The listing builds one solid part. Answer for the finished solid, in the listing's coordinates (mm). A direction names the side the tool comes from. Coordinates: 2 decimals unless noted, no trailing zeros. Loops run counter-clockwise (first coordinate to the right, second up) from the corner with the lowest first, then second, coordinate; pieces in that order, holes last. Notation, with made-up numbers: M -33.75,-23 L -29.75,-23 A21 cw -29.75,0 Z; hole C 20.25,-39 d10. An arc over 180 degrees is marked long. Return JSON: item names as keys, results as strings. Group by question number.
1. Section C-C (z = 16) is taken. Write down the section's boundary in (x, y), then the cut area to 3 significant figures.
2. Straight lines are drawn through the part: L1, parallel to Z at x = 1, y = 3.25; L2, parallel to Y at x = 1.75, z = 5.5; L3, parallel to X at y = -1, z = 4. For each, find the intervals that lie inside material, in ascending order. Write a range as from..to.
3. Section A-A (y = 2) is taken. Write down the section's boundary in (x, z).
4. Section B-B (x = 0) is taken. Write down the section's boundary in (y, z), then the cut area to 3 significant figures.
5. Which of the six approach directions +Z, -Z, +X, -X, +Y, -Y give full straight-line access (tool end or side, diameter ignored) to faces 1 (the face through (-0.54, 2.44, 10.4)), 2 (the face through (5.19, 1.99, 1.48))?
6. Section D-D (y = -3.5) is taken. Write down the section's boundary in (x, z), then the cut area to 3 significant figures.
7. Given P1, Ø4, axis at y = -1.5, z = 7.5, coming from the +X side; P2, Ø2, axis at x = 0, z = 9, coming from the -Y side; P3, Ø3, axis at x = -4.5, z = 14, coming from the -Y side; P4, Ø5, axis at x = -3.5, y = 2.5, coming from the +Z side, each flat-ended and moving along its own axis, determine where each tip first touches the part or whether it passes through.
Autodesk Inventor part; units mm, degrees
ref_plane "YZ Plane" through (0, 0, 0) normal (1, 0, 0) x (0, 1, 0)
ref_plane "XZ Plane" through (0, 0, 0) normal (0, 1, 0) x (-1, 0, 0)
ref_plane "XY Plane" through (0, 0, 0) normal (0, 0, 1) x (1, 0, 0)
sketch "Sketch1" plane through (0, 0, 0) normal (0, 0, 1) x (1, 0, 0)
  line L0 (-6.33, 1.0622) -> (-2.2451, 6.013)
  line L1 (-2.2451, 6.013) -> (4.0849, 4.9508)
  line L2 (4.0849, 4.9508) -> (6.33, -1.0622)
  line L3 (6.33, -1.0622) -> (2.2451, -6.013)
  line L4 (2.2451, -6.013) -> (-4.0849, -4.9508)
  line L5 (-4.0849, -4.9508) -> (-6.33, 1.0622)
  point P0 (0, 0)
  point P1 (0, 0)
extrude "Extrusion1" add sketch "Sketch1" along normal blind 3
sketch "Sketch2" plane through (0, 0, 3) normal (0, 0, 1) x (1, 0, 0)
  circle A0 centre (0, 0) radius 2.5
  dimension "d2" = 5
extrude "Extrusion2" add sketch "Sketch2" along normal blind 15
thread "Thread1"
properties part number "finalnut"
Worked out:
{
 "1": {"outline": "C 0,0 d5", "area": "19.6 mm^2"},
 "2": {"L1": "0..3", "L2": "-1.79..1.79", "L3": "-2.29..2.29"},
 "3": {"outline": "M -5.56,0 L 5.19,0 L 5.19,3 L 1.5,3 L 1.5,18 L -1.5,18 L -1.5,3 L -5.56,3 Z"},
 "4": {"outline": "M -5.64,0 L 5.64,0 L 5.64,3 L 2.5,3 L 2.5,18 L -2.5,18 L -2.5,3 L -5.64,3 Z", "area": "109 mm^2"},
 "5": {"face 1": "+Z", "face 2": "+Z, -Z, +X, +Y"},
 "6": {"outline": "M -4.63,0 L 4.32,0 L 4.32,3 L -4.63,3 Z", "area": "26.8 mm^2"},
 "7": {"P1": "x = 2.5", "P2": "y = -2.5", "P3": "through", "P4": "z = 18"}
}
